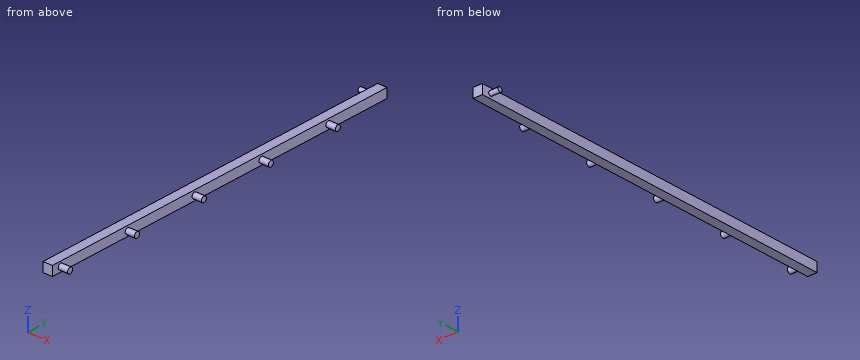
```python
from build123d import *

# Parameters (mm, degrees)
F0_W     = 1000
F0_H     = 25
F1_DEPTH = 25
F2_R     = 7.5
F3_DEPTH = 25
F4_R     = 6
F5_DEPTH = 25


with BuildPart() as f1:
    # F0 (on Right) → F1 (new body)
    with BuildSketch(Plane.YZ):
        Rectangle(F0_W, F0_H)
    extrude(amount=F1_DEPTH)

    # F2 (on face) → F3 (join)
    with BuildSketch(Plane.YZ.offset(25)):
        with Locations((-475, 0)):
            Circle(F2_R)
        with Locations((-275, 0)):
            Circle(F2_R)
        with Locations((-75, 0)):
            Circle(F2_R)
        with Locations((125, 0)):
            Circle(F2_R)
        with Locations((325, 0)):
            Circle(F2_R)
    extrude(amount=F3_DEPTH)

    # F4 (on face) → F5 (join)
    with BuildSketch(Plane(origin=(0, 0, 0), x_dir=(0, -1, 0), z_dir=(-1, 0, 0))):
        with Locations((-475, 0)):
            Circle(F4_R)
    extrude(amount=F5_DEPTH)


solid = f1.part
```
Verification items for the finished model (mm, model axes). Give positions to 0.01 mm unless a question says otherwise; leave off trailing zeros. Order: outer loops, then holes, each group sorted by start corner. A loop starts at its lowest first (then second) coordinate and runs counter-clockwise, first axis right, second up. Notation, with made-up numbers: M -5.75,51.25 L 30.25,51.25 A10 cw 30.25,68.25 Z; hole C -25.5,8.5 d5. An arc over 180 degrees is marked long. Return JSON: item names as keys, results as strings. Group by question number.
1) Scan lines: line 1 (Y direction, x = 42.5, z = 4); line 2 (Y direction, x = 41, z = -2); line 3 (X direction, y = 455, z = 3). Record each from-to range of solid material in increasing order.
2) Go/stop test with flat-tipped pins: pin 1 Ø6 at (y, z) = (-52, 3.5) entering from +X; pin 2 Ø8 at (x, z) = (-15.5, 9.5) entering from -Y; pin 3 Ø12.5 at (y, z) = (170, 4) entering from -X. Record where each tip stops, or that it passes through.
3) Section check C-C on x = -12. Record the cut outline in (y, z), and give its area (3 significant figures).
4) Section check B-B on y = 178. Record the cut outline in (x, z), and give its area (3 significant figures).
5) Section check A-A on x = 40.5. Record the cut outline in (y, z), and give its area (3 significant figures).
Answer block:
{
 "1": {"line 1": "y = -481.34 to -468.66, -281.34 to -268.66, -81.34 to -68.66, 118.66 to 131.34, 318.66 to 331.34", "line 2": "y = -482.23 to -467.77, -282.23 to -267.77, -82.23 to -67.77, 117.77 to 132.23, 317.77 to 332.23", "line 3": "x = 0 to 25"},
 "2": {"pin 1": "stops at x = 25", "pin 2": "stops at y = 472.6", "pin 3": "stops at x = 0"},
 "3": {"outline": "C 475,0 d12", "area": "113 mm^2"},
 "4": {"outline": "M 0,-12.5 L 25,-12.5 L 25,12.5 L 0,12.5 Z", "area": "625 mm^2"},
 "5": {"outline": "C -475,0 d15; C -275,0 d15; C -75,0 d15; C 125,0 d15; C 325,0 d15", "area": "884 mm^2"}
}
